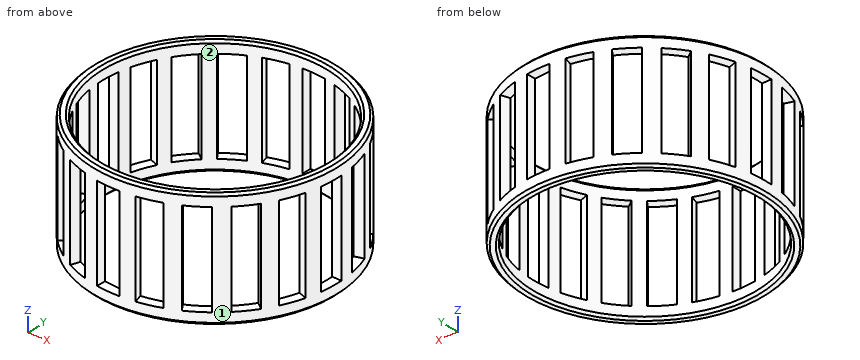
from build123d import *

# Parameters (mm, degrees)
ESQUISSE1_R                  = 26
ESQUISSE1_R_2                = 24
BASE_EXTRUSION_DEPTH         = 25
ENL_V_MAT_EXTRU_1_REACH      = 46.463
ESQUISSE2_W                  = 5
ESQUISSE2_H                  = 20
R_P_TITION_CIRCULAIRE2_COUNT = 20
CHANFREIN1_SIZE              = 0.5


with BuildPart() as part:
    # Esquisse1 → Base-Extrusion (new body)
    with BuildSketch(Plane.XY):
        Circle(ESQUISSE1_R)
        Circle(ESQUISSE1_R_2, mode=Mode.SUBTRACT)
    extrude(amount=BASE_EXTRUSION_DEPTH)

    # Esquisse2 → Enlèv. mat.-Extru.1 (cut, up to next)
    with BuildSketch(Plane(origin=(0, 0, 0), x_dir=(1, 0, 0), z_dir=(0, 1, 0)), mode=Mode.PRIVATE) as enl_v_mat_extru_1_sk1:
        with Locations((-0.75, -12.5)):
            Rectangle(ESQUISSE2_W, ESQUISSE2_H)
    enl_v_mat_extru_1_tool1 = extrude(enl_v_mat_extru_1_sk1.sketch, amount=-ENL_V_MAT_EXTRU_1_REACH, mode=Mode.PRIVATE) & part.part
    enl_v_mat_extru_1 = enl_v_mat_extru_1_tool1.solids().sort_by_distance((-0.75, 0, 12.5))[0]
    add(enl_v_mat_extru_1, mode=Mode.SUBTRACT)

    # Répétition circulaire2: Enlèv. mat.-Extru.1 ×20 about axis
    r_p_tition_circulaire2_axis = Axis((0, 0, 75), (0, 0, -1))
    for i in range(1, R_P_TITION_CIRCULAIRE2_COUNT):
        add(enl_v_mat_extru_1.rotate(r_p_tition_circulaire2_axis, i * 360 / R_P_TITION_CIRCULAIRE2_COUNT), mode=Mode.SUBTRACT)

    # Chanfrein1
    chanfrein1_edges = [part.edges().sort_by_distance(p)[0] for p in [
        (-26, 0, 25),
        (-26, 0, 0),
        (-24, 0, 25),
        (-24, 0, 0),
    ]]
    chamfer(chanfrein1_edges, length=CHANFREIN1_SIZE)


solid = part.part
The listing builds one solid part. Answer for the finished solid, in the listing's coordinates (mm). Face numbers are marked on the shaded views. Give positions to 0.01 mm unless a question says otherwise; leave off trailing zeros. Loops run counter-clockwise (first coordinate to the right, second up) from the corner with the lowest first, then second, coordinate; pieces in that order, holes last. Notation, with made-up numbers: M 38.25,7.25 L 88.25,7.25 A16 cw 88.25,13.25 Z; hole C 57.25,70.25 d11. An arc over 180 degrees is marked long. Answer as CSV lines item,"result".
Item 1: The part is cut by section A-A (y = 0). Give the vertices of the cut face in (x, z), and give its area (3 significant figures).
Values follow:
outline,"M -26,0.5 L -25.5,0 L -24.5,0 L -24,0.5 L -24,2.5 L -26,2.5 Z; M -26,22.5 L -24,22.5 L -24,24.5 L -24.5,25 L -25.5,25 L -26,24.5 Z; M 24,0.5 L 24.5,0 L 25.5,0 L 26,0.5 L 26,2.5 L 24,2.5 Z; M 24,22.5 L 26,22.5 L 26,24.5 L 25.5,25 L 24.5,25 L 24,24.5 Z"
area,"19.0 mm^2"
Item 2: Straight lines are drawn through the part: line 1 along Y through (x, z) = (-24, 10.25); line 2 along X through (y, z) = (18, 7); line 3 along X through (y, z) = (22, 19.75). For each, find the intervals that lie inside material, in ascending order. Write a range as [from, to].
Values follow:
line 1,"y = [-10, -9.64], [-4.38, -1.75], [3.25, 5.96]"
line 2,"x = [-18.76, -15.87], [17.09, 18.76]"
line 3,"x = [-11.97, -9.59], [10.57, 13.82]"
Item 3: The part is cut by section C-C (z = 3.5). Give the number of separate pieces and of enclosed holes in the cut face, and give its area (3 significant figures).
Values follow:
separate pieces,"20"
enclosed holes,"0"
area,"114 mm^2"
Item 4: The mould has two halves that part along Y. Classify the marked faces 1 and 2: released by +Y, released by -Y, zero draft, split by the parting line, or undercut.
Values follow:
face 1,"split by the parting line"
face 2,"undercut"
Item 5: Given pin 1 Ø1.5 at (y, z) = (-2, 6) entering from -X; pin 2 Ø5 at (x, z) = (6.5, 14) entering from +Y; pin 3 Ø1.6 at (y, z) = (-24.5, 8.5) entering from -X, each flat-ended and moving along its own axis, determine where each tip first touches the part or whether it passes through.
Values follow:
pin 1,"stops at x = -25.94"
pin 2,"stops at y = 25.69"
pin 3,"stops at x = -6.35"
